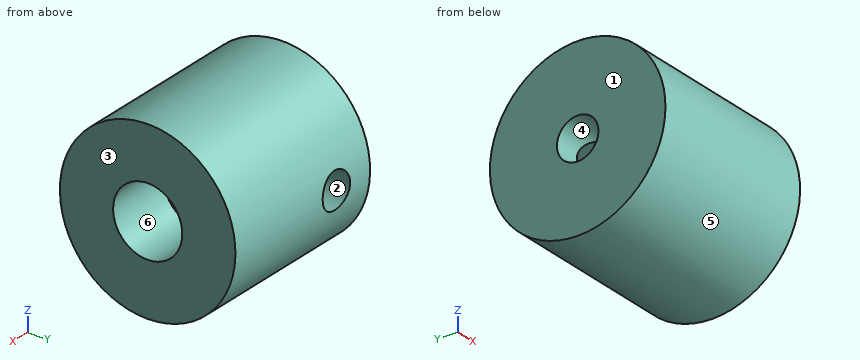
```python
from build123d import *

# Parameters (mm, degrees)
SKETCH1_R           = 12.7
BOSS_EXTRUDE1_DEPTH = 25.4
SKETCH2_R           = 3
CUT_EXTRUDE1_DEPTH  = 9.525
SKETCH3_R           = 5
CUT_EXTRUDE2_DEPTH  = 9.525


with BuildPart() as part:
    # Sketch1 → Boss-Extrude1 (new body)
    with BuildSketch(Plane(origin=(0, 0, 0), x_dir=(0, 0, -1), z_dir=(1, 0, 0))):
        Circle(SKETCH1_R)
    extrude(amount=BOSS_EXTRUDE1_DEPTH)

    # Sketch2 → Cut-Extrude1 (cut)
    with BuildSketch(Plane.ZY):
        Circle(SKETCH2_R)
    extrude(amount=-CUT_EXTRUDE1_DEPTH, mode=Mode.SUBTRACT)

    # Sketch7 → #6 (0.204) Diameter Hole1 (revolve, cut)
    with BuildSketch(Plane(origin=(6.35, 0, 0), x_dir=(0, 0, -1), z_dir=(1, 0, 0))):
        Polygon((0, 0), (0, 16.288709692), (2.5908, 14.732), (2.5908, 0), align=None)
    revolve(axis=Axis((6.35, -6.35, 0), (0, 1, 0)), mode=Mode.SUBTRACT)

    # Sketch3 → Cut-Extrude2 (cut)
    with BuildSketch(Plane(origin=(25.4, 0, 0), x_dir=(0, 0, -1), z_dir=(1, 0, 0))):
        Circle(SKETCH3_R)
    extrude(amount=-CUT_EXTRUDE2_DEPTH, mode=Mode.SUBTRACT)


solid = part.part
```
Read the model definition and answer for the solid it produces. Units are mm, in the model's axes. Face numbers are marked on the shaded views. A direction names the side the tool comes from. Round coordinates to 2 decimals unless told otherwise and drop trailing zeros. Write each loop counter-clockwise with the first axis right and the second up, starting at its lowest first coordinate (ties: lowest second). Pieces come first, ordered by that corner, then holes. Notation, with made-up numbers: (-31.75, 14) - (-4.75, 14) arc R21 ccw to (-4.75, 44) - close; hole circle Ø8 at (34, 34). An arc over 180 degrees is marked (long way). One line per item, written item: value.
Q1. Straight lines are drawn through the part: line 1 (X direction, y = 7.25, z = 0); line 2 (Y direction, x = 2, z = 0); line 3 (X direction, y = 0, z = 1.5) (3 decimals). For each, find the intervals that lie inside material, in ascending order. Write a range as from..to.
The answers:
line 1: x = 0..3.76, 8.94..25.4
line 2: y = -12.7..-3, 3..12.7
line 3: x = 9.525..15.875
Q2. Find section B-B (y = 0). Determine the outline of the cut face in (x, z) (3 decimals).
The answers:
outline: (0, -12.7) - (25.4, -12.7) - (25.4, -5) - (15.875, -5) - (15.875, 5) - (25.4, 5) - (25.4, 12.7) - (0, 12.7) - (0, 3) - (9.525, 3) - (9.525, -3) - (0, -3) - close
Q3. Find section A-A (z = 0). Determine the outline of the cut face in (x, y) (3 decimals), and give its area (3 significant figures).
The answers:
outline: (0, -12.7) - (25.4, -12.7) - (25.4, -5) - (15.875, -5) - (15.875, 5) - (25.4, 5) - (25.4, 12.7) - (8.941, 12.7) - (8.941, 3) - (9.525, 3) - (9.525, -3) - (0, -3) - close; (0, 3) - (3.759, 3) - (3.759, 12.7) - (0, 12.7) - close
area: 442 mm2
Q4. Each of these flat-tipped pins is pushed along its axis until it touches: P1, Ø1.5, axis at x = 3.5, z = -1, coming from the -Y side; P2, Ø1.5, axis at x = 20.5, y = 3.5, coming from the +Z side; P3, Ø3, axis at y = 2, z = 0, coming from the +X side (3 decimals). Where does it stop, or does it pass through?
The answers:
P1: stops at y = -12.7
P2: stops at z = 12.4
P3: stops at x = 15.875
Q5. Find section D-D (z = -11). Determine the outline of the cut face in (x, y).
The answers:
outline: (0, -6.35) - (25.4, -6.35) - (25.4, 6.35) - (0, 6.35) - close
Q6. Which of the six approach directions +Z, -Z, +X, -X, +Y, -Y give full straight-line access (tool end or side, diameter ignored) to the marked faces 1 and 2?
The answers:
face 1: +Z, -Z, -X, +Y, -Y
face 2: +Y
Q7. For a pull along Y with two mould halves and no side action, classify the marked faces 3, 4, 5 and 6 as pulls with the +Y half, pulls with the -Y half, needs draft (parallel to the pull), parting line crosses it, or undercut.
The answers:
face 3: needs draft
face 4: undercut
face 5: parting line crosses it
face 6: undercut
Q8. Find section C-C (x = 19.5). Determine the outline of the cut face in (y, z), and give its area (3 significant figures).
The answers:
outline: circle Ø25.4 at (0, 0); hole circle Ø10 at (0, 0)
area: 428 mm2
